from build123d import *

# Parameters (mm, degrees)
F0_W     = 127
F0_H     = 127
F0_R     = 38.1
F1_DEPTH = 127
F2_DEPTH = 165.1
F3_R     = 6.35
F4_SIZE  = 6.34999


# Not quite as in the source:
# - a fillet or chamfer is up to 0.001 mm smaller than in the source, because OpenCascade refuses the exact size


with BuildPart() as f1:
    # F0 (on Top) → F1 (new body)
    with BuildSketch(Plane.XY):
        Rectangle(F0_W, F0_H)
        Circle(F0_R, mode=Mode.SUBTRACT)
        Circle(F0_R)
    extrude(amount=-F1_DEPTH)

    # F0 (on Top) → F2 (join)
    with BuildSketch(Plane.XY):
        Circle(F0_R)
    extrude(amount=F2_DEPTH)

    # F3
    f3_edges = [f1.edges().sort_by_distance(p)[0] for p in [
        (-63.5, -63.5, -63.5),
        (63.5, -63.5, -63.5),
        (63.5, 63.5, -63.5),
        (-63.5, 63.5, -63.5),
    ]]
    fillet(f3_edges, radius=F3_R)

    # F4 (size 6.35 in the source; OpenCascade refuses exactly that, so slightly less here)
    f4_edges = [f1.edges().sort_by_distance(p)[0] for p in [
        (0, -63.5, 0),
    ]]
    chamfer(f4_edges, length=F4_SIZE)


solid = f1.part
Verification items for the finished model (mm, model axes). A direction names the side the tool comes from. Round coordinates to 2 decimals unless told otherwise and drop trailing zeros. Loops run counter-clockwise (first coordinate to the right, second up) from the corner with the lowest first, then second, coordinate; pieces in that order, holes last. Notation, with made-up numbers: (60.25, 81) - (101.25, 81) arc R17 cw to (101.25, 91) - close; hole circle Ø4 at (83.25, -18). An arc over 180 degrees is marked (long way). Write item = value, one per line.
Q1. Mould release check, pull along Y, two halves, no side actions. Record for faces 1 (the flat face through (63.5, -1, -66)), 2 (the cylindrical face through (-61.69, -61.59, -67.52)), 3 (the cylindrical face through (-30.235, -23.183, 81.394)), 4 (the conical face through (59.45, 59.4, -3.22)): +Y half, -Y half, draft (parallel to the pull), parting line (faces both ways), or undercut.
Here are the results:
face_1 = draft
face_2 = -Y half
face_3 = parting line
face_4 = +Y half
Q2. Sectioned sample at C-C on z = 14. Record the boundary of the cut face in (x, y).
Here are the results:
outline = circle Ø76.2 at (0, 0)
Q3. Material ranges on L1, parallel to Z at x = -55, y = 22; L2, parallel to Y at x = 1, z = 114; L3, parallel to Y at x = -28, z = 95, recorded low to high.
Here are the results:
L1 = -127 to 0
L2 = -38.09 to 38.09
L3 = -25.84 to 25.84
Q4. Tool access check on faces 5 (the flat face through (-39, 1, 0)), 6 (the cylindrical face through (-61.69, 61.59, -67.52)). Record the directions out of +Z, -Z, +X, -X, +Y, -Y that give a thin tool (end or side, any length) a straight path to the whole face; none if there is none.
Here are the results:
face_5 = +Z
face_6 = +Z, -Z, -X, +Y
Q5. Sectioned sample at A-A on y = 0. Record the boundary of the cut face in (x, z).
Here are the results:
outline = (-63.5, -127) - (63.5, -127) - (63.5, -6.35) - (57.15, 0) - (38.1, 0) - (38.1, 165.1) - (-38.1, 165.1) - (-38.1, 0) - (-57.15, 0) - (-63.5, -6.35) - close
Q6. Depth check by flat-ended pin: pin 1 (1.5 mm diameter, centred on y = 30, z = 77.5, fed in from +X); pin 2 (1 mm diameter, centred on x = -4.5, z = 33.5, fed in from -Y); pin 3 (3 mm diameter, centred on y = -5, z = 90.5, fed in from -X). Enter the tip coordinate at first touch or a pass-through.
Here are the results:
pin_1 = 24.41
pin_2 = -37.89
pin_3 = -37.94
Q7. Sectioned sample at D-D on y = 50. Record the boundary of the cut face in (x, z).
Here are the results:
outline = (-63.5, -127) - (63.5, -127) - (63.5, -6.35) - (57.15, 0) - (-57.15, 0) - (-63.5, -6.35) - close
